The model under review builds one solid part; all positions refer to its coordinate system, in mm. Give positions to 0.01 mm unless a question says otherwise; leave off trailing zeros. Loops run counter-clockwise (first coordinate to the right, second up) from the corner with the lowest first, then second, coordinate; pieces in that order, holes last. Notation, with made-up numbers: (62.25, -10) - (116.25, -10) arc R24 cw to (116.25, 7) - close; hole circle Ø2 at (28.25, 80). An arc over 180 degrees is marked (long way). Answer as a JSON object with one key per item and string values.
from build123d import *

# Parameters (mm, degrees)
SKETCH_1_R      = 50
SKETCH_1_R_2    = 43.3
EXTRUDE_1_DEPTH = 2
SKETCH_2_R      = 1.6
EXTRUDE_2_DEPTH = 2
FILLET_1_R      = 5


with BuildPart() as part:
    # 草图1 → 凸台-拉伸1 (new body)
    with BuildSketch(Plane(origin=(0, 0, 0), x_dir=(1, 0, 0), z_dir=(0, 1, 0))):
        with Locations(Location((0, 0, 0), (0, 0, 270))):
            Circle(SKETCH_1_R)
        with Locations(Location((0, 0, 0), (0, 0, 270))):
            Circle(SKETCH_1_R_2, mode=Mode.SUBTRACT)
    extrude(amount=EXTRUDE_1_DEPTH)

    # 草图2 → 凸台-拉伸2 (add)
    # profile 1 of 4: a face of its own
    with BuildSketch(Plane(origin=(0, 2, 0), x_dir=(1, 0, 0), z_dir=(0, 1, 0))):
        with BuildLine():
            Line((47.683371348, 4), (47.683371348, -4))
            Line((47.683371348, -4), (61, -4))
            ThreePointArc((61, -4), (65, 0), (61, 4))
            Line((61, 4), (47.683371348, 4))
        make_face()
        with Locations(Location((61, 0, 0), (0, 0, 270))):
            Circle(SKETCH_2_R, mode=Mode.SUBTRACT)
    # profile 2 of 4: a face of its own
    with BuildSketch(Plane(origin=(0, 2, 0), x_dir=(1, 0, 0), z_dir=(0, 1, 0))):
        with BuildLine():
            Line((-4, -61), (-4, -47.683371348))
            Line((-4, -47.683371348), (4, -47.683371348))
            Line((4, -47.683371348), (4, -61))
            ThreePointArc((4, -61), (0, -65), (-4, -61))
        make_face()
        with Locations(Location((0, -61, 0), (0, 0, 270))):
            Circle(SKETCH_2_R, mode=Mode.SUBTRACT)
    # profile 3 of 4: a face of its own
    with BuildSketch(Plane(origin=(0, 2, 0), x_dir=(1, 0, 0), z_dir=(0, 1, 0))):
        with BuildLine():
            Line((-61, 4), (-47.683371348, 4))
            Line((-47.683371348, 4), (-47.683371348, -4))
            Line((-47.683371348, -4), (-61, -4))
            ThreePointArc((-61, -4), (-65, 0), (-61, 4))
        make_face()
        with Locations(Location((-61, 0, 0), (0, 0, 270))):
            Circle(SKETCH_2_R, mode=Mode.SUBTRACT)
    # profile 4 of 4: a face of its own
    with BuildSketch(Plane(origin=(0, 2, 0), x_dir=(1, 0, 0), z_dir=(0, 1, 0))):
        with BuildLine():
            Line((4, 61), (4, 47.683371348))
            Line((4, 47.683371348), (-4, 47.683371348))
            Line((-4, 47.683371348), (-4, 61))
            ThreePointArc((-4, 61), (0, 65), (4, 61))
        make_face()
        with Locations(Location((0, 61, 0), (0, 0, 270))):
            Circle(SKETCH_2_R, mode=Mode.SUBTRACT)
    extrude(amount=-EXTRUDE_2_DEPTH)

    # 圆角1
    fillet_1_edges = [part.edges().sort_by_distance(p)[0] for p in [
        (49.839743178, 1, -4),
        (49.839743178, 1, 4),
        (-4, 1, 49.839743178),
        (4, 1, 49.839743178),
        (-49.839743178, 1, -4),
        (-49.839743178, 1, 4),
        (4, 1, -49.839743178),
        (-4, 1, -49.839743178),
    ]]
    fillet(fillet_1_edges, radius=FILLET_1_R)


solid = part.part
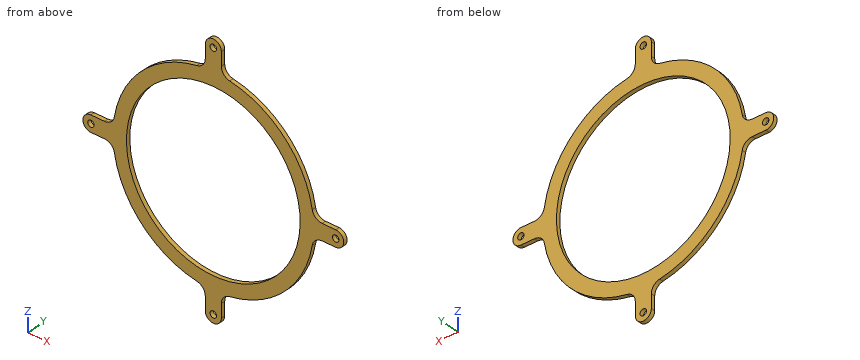
Q1. Clearance check with flat-ended pins moving along their axes: pin 1 Ø3 at (x, z) = (-61, 0) entering from -Y; pin 2 Ø1 at (y, z) = (1, 59) entering from -X; pin 3 Ø0.6 at (x, y) = (-57, 1.5) entering from -Z; pin 4 Ø0.6 at (y, z) = (1, 58.5) entering from +X. State where each tip first meets the part, or that it passes through.
Results:
{"pin 1": "passes through", "pin 2": "stops at x = -4", "pin 3": "stops at z = -4", "pin 4": "stops at x = 4"}
Q2. Consider section A-A, the plane y = 0.85. State how many separate pieces and enclosed holes the cut face has, plus the area to 3 significant figures.
Results:
{"separate pieces": "1", "enclosed holes": "5", "area": "2,420 mm^2"}
Q3. To check wall thickness, follow probe 1 along X at (y, z) = (0.85, 0); probe 2 along X at (y, z) = (0.75, -61); probe 3 along X at (y, z) = (1.4, -15). State the ranges of each line that lie inside material, in increasing order. Write a range as [from, to].
Results:
{"probe 1": "x = [-65, -62.6], [-59.4, -43.3], [43.3, 59.4], [62.6, 65]", "probe 2": "x = [-4, -1.6], [1.6, 4]", "probe 3": "x = [-47.7, -40.62], [40.62, 47.7]"}
Q4. Consider section C-C, the plane z = 0. State the section outline as (x, y) points, plus the area to 3 significant figures.
Results:
{"outline": "(-65, 0) - (-62.6, 0) - (-62.6, 2) - (-65, 2) - close; (-59.4, 0) - (-43.3, 0) - (-43.3, 2) - (-59.4, 2) - close; (43.3, 0) - (59.4, 0) - (59.4, 2) - (43.3, 2) - close; (62.6, 0) - (65, 0) - (65, 2) - (62.6, 2) - close", "area": "74.0 mm^2"}
Q5. Consider section B-B, the plane x = 0. State the section outline as (y, z) points, plus the area to 3 significant figures.
Results:
{"outline": "(0, -65) - (2, -65) - (2, -62.6) - (0, -62.6) - close; (0, -59.4) - (2, -59.4) - (2, -43.3) - (0, -43.3) - close; (0, 43.3) - (2, 43.3) - (2, 59.4) - (0, 59.4) - close; (0, 62.6) - (2, 62.6) - (2, 65) - (0, 65) - close", "area": "74.0 mm^2"}
Q6. Consider section D-D, the plane x = -41.5. State the section outline as (y, z) points.
Results:
{"outline": "(0, -27.89) - (2, -27.89) - (2, -12.35) - (0, -12.35) - close; (0, 12.35) - (2, 12.35) - (2, 27.89) - (0, 27.89) - close"}
